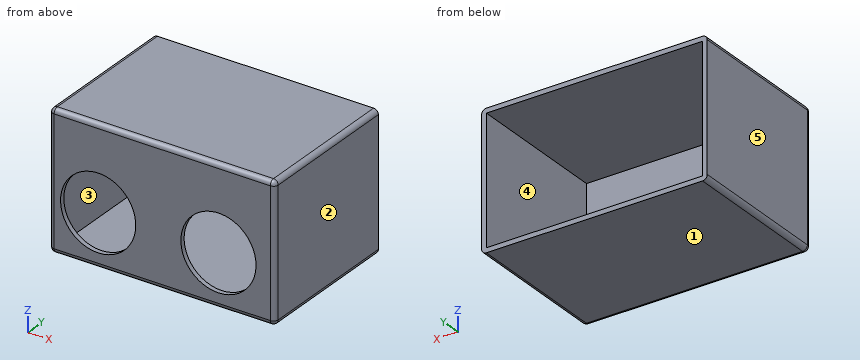
```python
from build123d import *

# Parameters (mm, degrees)
SKETCH_1_W          = 48
SKETCH_1_H          = 29
EXTRUDE_1_DEPTH     = 32
SKETCH_4_W          = 46
SKETCH_4_H          = 27
CUT_EXTRUDE_1_DEPTH = 31
FILLET_1_R          = 1
SKETCH_5_R          = 8
CUT_EXTRUDE_2_DEPTH = 1


with BuildPart() as part:
    # ｽｹｯﾁ1 → ﾎﾞｽ - 押し出し1 (new body)
    with BuildSketch(Plane(origin=(0, 0, 0), x_dir=(1, 0, 0), z_dir=(0, 1, 0))):
        with Locations((-8.709727642, 40.94775)):
            Rectangle(SKETCH_1_W, SKETCH_1_H)
    extrude(amount=EXTRUDE_1_DEPTH)

    # ｽｹｯﾁ4 → ｶｯﾄ - 押し出し1 (cut)
    with BuildSketch(Plane(origin=(0, 32, 0), x_dir=(1, 0, 0), z_dir=(0, 1, 0))):
        with Locations((-8.709727642, 40.94775)):
            Rectangle(SKETCH_4_W, SKETCH_4_H)
    extrude(amount=-CUT_EXTRUDE_1_DEPTH, mode=Mode.SUBTRACT)

    # ﾌｨﾚｯﾄ1
    fillet_1_edges = [part.edges().sort_by_distance(p)[0] for p in [
        (-8.709727642, 0, -55.44775),
        (15.290272358, 0, -40.94775),
        (-8.709727642, 0, -26.44775),
        (-32.709727642, 0, -40.94775),
        (-32.709727642, 16, -55.44775),
        (15.290272358, 16, -55.44775),
        (15.290272358, 16, -26.44775),
        (-32.709727642, 16, -26.44775),
    ]]
    fillet(fillet_1_edges, radius=FILLET_1_R)

    # ｽｹｯﾁ5 → ｶｯﾄ - 押し出し2 (cut)
    with BuildSketch(Plane(origin=(0, 0, 0), x_dir=(-1, 0, 0), z_dir=(0, -1, 0))):
        with Locations(Location((-3.260272358, 44.346563504, 0), (0, 0, 90))):
            Circle(SKETCH_5_R)
        with Locations(Location((22.339727642, 44.346653581, 0), (0, 0, 90))):
            Circle(SKETCH_5_R)
    extrude(amount=-CUT_EXTRUDE_2_DEPTH, mode=Mode.SUBTRACT)


solid = part.part
```
Input: part model. Units: mm. Frame: model coordinates. Face numbers are marked on the shaded views. A direction names the side the tool comes from. Coordinates: 2 decimals unless noted, no trailing zeros. Loops run counter-clockwise (first coordinate to the right, second up) from the corner with the lowest first, then second, coordinate; pieces in that order, holes last.
Q1. Section A-A, the plane y = 18. Return the cut outline in (x, z).
Results are:
outline: (-32.71, -54.45) arc R1 ccw to (-31.71, -55.45) - (14.29, -55.45) arc R1 ccw to (15.29, -54.45) - (15.29, -27.45) arc R1 ccw to (14.29, -26.45) - (-31.71, -26.45) arc R1 ccw to (-32.71, -27.45) - close; hole (-31.71, -54.45) - (14.29, -54.45) - (14.29, -27.45) - (-31.71, -27.45) - close
Q2. Line query: line 1 along Z through (x, y) = (-25.5, 18); line 2 along X through (y, z) = (7, -31.75); line 3 along Y through (x, z) = (-21, -35). Output: solid intervals per line, ascending.
Results are:
line 1: z = -55.45 to -54.45, -27.45 to -26.45
line 2: x = -32.71 to -31.71, 14.29 to 15.29
line 3: y = 0 to 1
Q3. Section C-C, the plane x = -25. Return the cut outline in (y, z).
Results are:
outline: (0, -54.45) arc R1 ccw to (1, -55.45) - (32, -55.45) - (32, -54.45) - (1, -54.45) - (1, -51.89) - (0, -51.89) - close; (0, -36.8) - (1, -36.8) - (1, -27.45) - (32, -27.45) - (32, -26.45) - (1, -26.45) arc R1 ccw to (0, -27.45) - close
Q4. Section D-D, the plane z = -30.75. Return the cut outline in (x, y), and give its area (3 significant figures).
Results are:
outline: (-32.71, 1) arc R1 ccw to (-31.71, 0) - (14.29, 0) arc R1 ccw to (15.29, 1) - (15.29, 32) - (14.29, 32) - (14.29, 1) - (-31.71, 1) - (-31.71, 32) - (-32.71, 32) - close
area: 110 mm2
Q5. Mould query, pull axis X, two halves, no side actions, for the marked faces 1, 2 and 3. Classes: +X half, -X half, draft (parallel to the pull), parting line (faces both ways), or undercut.
Results are:
face 1: draft
face 2: +X half
face 3: undercut
Q6. Set-up query: the marked faces 4 and 5. Return all of +Z, -Z, +X, -X, +Y, -Y with unobstructed straight access to the full face (end or side cutting, diameter ignored); none if empty.
Results are:
face 4: +Y
face 5: +Z, -Z, -X, +Y, -Y
Q7. Contact query for a flat-ended pin moving along its axis: pin 1 (3 mm diameter, centred on x = -5, z = -34, fed in from +Y). Output: stop coordinate, or through.
Results are:
pin 1: stops at y = 1
Q8. Section B-B, the plane z = -48.75. Return the cut outline in (x, y), and give its area (3 significant figures).
Results are:
outline: (-32.71, 1) arc R1 ccw to (-31.71, 0) - (-29.02, 0) - (-29.02, 1) - (-31.71, 1) - (-31.71, 32) - (-32.71, 32) - close; (-15.66, 0) - (-3.42, 0) - (-3.42, 1) - (-15.66, 1) - close; (9.94, 0) - (14.29, 0) arc R1 ccw to (15.29, 1) - (15.29, 32) - (14.29, 32) - (14.29, 1) - (9.94, 1) - close
area: 82.9 mm2
